The model under review builds one solid part; all positions refer to its coordinate system, in mm. A direction names the side the tool comes from. Coordinates: 2 decimals unless noted, no trailing zeros. Order: outer loops, then holes, each group sorted by start corner. A loop starts at its lowest first (then second) coordinate and runs counter-clockwise, first axis right, second up. Notation, with made-up numbers: M 24,-31 L 71,-31 A13 ccw 71,-21 Z; hole C 46.5,62.25 d5. An arc over 180 degrees is marked long. Answer as CSV lines item,"result". Start each with the question number.
Q1. The part is to be moulded in two halves that separate along X. For faces 1 (the face through (-36.557, 8.507, 15.291)), 2 (the face through (8.766, 0.126, 101.404)), 3 (the face through (3, 0, 125.39)), say which applies: +X half, -X half, draft (parallel to the pull), parting line (faces both ways), or undercut.
Q2. Wall thickness on L1, parallel to Y at x = -21.5, z = 84; L2, parallel to Z at x = -37.5, y = 6.5; L3, parallel to X at y = 8.75, z = 28: over which ranges is each line inside the solid? List them lowest first. Write a range as [from, to].
Q3. Consider section B-B on x = 9. State how many separate pieces and enclosed holes the cut face has, and give its area (3 significant figures).
Q4. Consider section A-A on z = 29.5. Write out the cut boundary in (x, y).
Q5. Machinability: for faces 4 (the face through (1.248, 0.126, 65.957)), 5 (the face through (-27.87, -8.51, 44.64)), 6 (the face through (8.766, 0.126, 107.404)), 7 (the face through (-25, 11, 84)), which of the approach directions +Z, -Z, +X, -X, +Y, -Y give a long, thin tool a straight path to every point of the face, cutting with its end or side? Answer none if there is none.
Q6. For P1, Ø0.9, axis at x = -25.5, z = 84.5, coming from the +Y side; P2, Ø2, axis at y = 2.5, z = 93, coming from the +X side; P3, Ø6, axis at y = 4, z = 64, coming from the -X side, all flat-tipped, find the tip position at first contact; note any pin that passes through.
from build123d import *

# Parameters (mm, degrees)
BOSS_EXTRUDE1_DEPTH = 9
FILLET1_R           = 6
FILLET2_R           = 4
BOSS_EXTRUDE2_DEPTH = 18
LPATTERN1_COUNT     = 6
LPATTERN1_PITCH     = 6
CUT_EXTRUDE1_DEPTH  = 19
CUT_EXTRUDE2_DEPTH  = 8
SKETCH5_R           = 1.5
CUT_EXTRUDE3_DEPTH  = 19
SKETCH6_R           = 1.75
BOSS_EXTRUDE3_DEPTH = 3
SKETCH7_R           = 1.55
CUT_EXTRUDE4_DEPTH  = 1
SKETCH8_R           = 1.55
CUT_EXTRUDE5_DEPTH  = 1
CUT_EXTRUDE7_DEPTH  = 1


with BuildPart() as part:
    # Sketch1 → Boss-Extrude1 (new body, symmetric)
    with BuildSketch(Plane(origin=(0, 0, 0), x_dir=(1, 0, 0), z_dir=(0, 1, 0))):
        with BuildLine():
            Line((-12.33246069, -71), (-19.816764537, -74.012394232))
            Line((-19.816764537, -74.012394232), (-26.247607485, -76.600775811))
            Line((-26.247607485, -76.600775811), (-30.167039554, -85.800669955))
            Line((-30.167039554, -85.800669955), (-18.831549927, -92.165155394))
            Line((-18.831549927, -92.165155394), (-4.262261991, -118.389873678))
            Line((-4.262261991, -118.389873678), (-4.262261991, -125.389873678))
            Line((-4.262261991, -125.389873678), (6.737738009, -125.389873678))
            Line((6.737738009, -125.389873678), (6.737738009, -75.389873678))
            Line((6.737738009, -75.389873678), (13.808805821, -68.318805866))
            ThreePointArc((13.808805821, -68.318805866), (12.667091661, -59.910685459), (4.258971254, -61.052399619))
            Line((4.258971254, -61.052399619), (-1.849045895, -71))
            Line((-1.849045895, -71), (-12.33246069, -71))
        make_face()
        Polygon((-12.33246069, -71), (-19.816764537, -74.012394232), (-45.953718322, -9.075042525), (-23.735626524, 0), align=None)
    extrude(amount=BOSS_EXTRUDE1_DEPTH, both=True)

    # Fillet1
    fillet1_edges = [part.edges().sort_by_distance(p)[0] for p in [
        (-45.953718322, 0, 9.075042525),
        (-23.735626524, 0, 0),
    ]]
    fillet(fillet1_edges, radius=FILLET1_R)

    # Fillet2
    fillet2_edges = [part.edges().sort_by_distance(p)[0] for p in [
        (-4.262261991, 0, 125.389873678),
        (-30.167039554, 0, 85.800669955),
        (-26.247607485, 0, 76.600775811),
    ]]
    fillet(fillet2_edges, radius=FILLET2_R)

    # Sketch2 → Boss-Extrude2 (add)
    with BuildSketch(Plane(origin=(0, 9, 0), x_dir=(1, 0, 0), z_dir=(0, 1, 0))):
        Polygon((6.737738009, -118.389873678), (6.737738009, -122.389873678), (10.737738009, -120.389873678), align=None)
    boss_extrude2 = extrude(amount=-BOSS_EXTRUDE2_DEPTH)

    # LPattern1: Boss-Extrude2 ×6
    with Locations(*[(0, 0, -i * LPATTERN1_PITCH) for i in range(1, LPATTERN1_COUNT)]):
        add(boss_extrude2)

    # Sketch3 → Cut-Extrude1 (cut, through all)
    with BuildSketch(Plane(origin=(0, 9, 0), x_dir=(1, 0, 0), z_dir=(0, 1, 0))):
        Polygon((4.039450666, -92.96261283), (-10.960549334, -92.96261283), (4.039450666, -117.96261283), align=None)
    extrude(amount=-CUT_EXTRUDE1_DEPTH, mode=Mode.SUBTRACT)

    # Sketch4 → Cut-Extrude2 (cut)
    with BuildSketch(Plane(origin=(-53.516863555, 0, 29.731590864), x_dir=(0.485642931, 0, 0.874157276), z_dir=(-0.874157276, 0, 0.485642931))):
        Polygon((78.421432088, 6), (78.421432088, -6), (96.421432088, -5.431048589), (96.421432088, 5.431048589), align=None)
    extrude(amount=-CUT_EXTRUDE2_DEPTH, mode=Mode.SUBTRACT)

    # Sketch5 → Cut-Extrude3 (cut, through all)
    with BuildSketch(Plane(origin=(0, 9, 0), x_dir=(1, 0, 0), z_dir=(0, 1, 0))):
        with Locations((-38.158783011, -12.372383774)):
            Circle(SKETCH5_R)
    extrude(amount=-CUT_EXTRUDE3_DEPTH, mode=Mode.SUBTRACT)

    # Sketch6 → Boss-Extrude3 (add)
    with BuildSketch(Plane(origin=(0, 9, 0), x_dir=(1, 0, 0), z_dir=(0, 1, 0))):
        with Locations((-25.081319154, -84.068763596)):
            Circle(SKETCH6_R)
        with Locations((9.033888537, -64.685602742)):
            Circle(SKETCH6_R)
    boss_extrude3 = extrude(amount=BOSS_EXTRUDE3_DEPTH)

    # Sketch7 → Cut-Extrude4 (cut)
    with BuildSketch(Plane(origin=(0, 12, 0), x_dir=(1, 0, 0), z_dir=(0, 1, 0))):
        with Locations((-25.081319154, -84.068763596)):
            Circle(SKETCH7_R)
    cut_extrude4 = extrude(amount=-CUT_EXTRUDE4_DEPTH, mode=Mode.SUBTRACT)

    # Sketch8 → Cut-Extrude5 (cut)
    with BuildSketch(Plane(origin=(0, 12, 0), x_dir=(1, 0, 0), z_dir=(0, 1, 0))):
        with Locations((9.033888537, -64.685602742)):
            Circle(SKETCH8_R)
    cut_extrude5 = extrude(amount=-CUT_EXTRUDE5_DEPTH, mode=Mode.SUBTRACT)

    # Sketch9 → Cut-Extrude7 (cut)
    with BuildSketch(Plane(origin=(0, 9, 0), x_dir=(1, 0, 0), z_dir=(0, 1, 0))):
        with BuildLine():
            Line((-34.306763605, -16.326309504), (-15.181058532, -69.865166146))
            ThreePointArc((-15.181058532, -69.865166146), (-16.229593753, -72.079184588), (-18.443612196, -71.030649368))
            Line((-18.443612196, -71.030649368), (-37.569317268, -17.491792726))
            ThreePointArc((-37.569317268, -17.491792726), (-36.520782048, -15.277774283), (-34.306763605, -16.326309504))
        make_face()
    cut_extrude7 = extrude(amount=-CUT_EXTRUDE7_DEPTH, mode=Mode.SUBTRACT)

    # Mirror1: Boss-Extrude3, Cut-Extrude4, Cut-Extrude5, Cut-Extrude7 across plane
    add(boss_extrude3.mirror(Plane.ZX))
    add(cut_extrude4.mirror(Plane.ZX), mode=Mode.SUBTRACT)
    add(cut_extrude5.mirror(Plane.ZX), mode=Mode.SUBTRACT)
    add(cut_extrude7.mirror(Plane.ZX), mode=Mode.SUBTRACT)


solid = part.part
Evaluation:
1,face 1,"undercut"
1,face 2,"+X half"
1,face 3,"draft"
2,L1,"y = [-9, 9]"
2,L2,"z = [5.62, 11.02], [13.72, 30.08]"
2,L3,"x = [-38.34, -33.82], [-30.14, -19.24]"
3,separate pieces,"7"
3,enclosed holes,"0"
3,area,"462 mm²"
4,outline,"M -37.73,-9 L -33.28,-9 L -33.28,-8 L -29.6,-8 L -29.6,-9 L -19,-9 L -19,9 L -29.6,9 L -29.6,8 L -33.28,8 L -33.28,9 L -37.73,9 Z"
5,face 4,"-Z, +Y, -Y"
5,face 5,"-Y"
5,face 6,"+X, +Y, -Y"
5,face 7,"+Y"
6,P1,"stops at y = 11"
6,P2,"stops at x = 7.52"
6,P3,"stops at x = -25.05"
